The model under review builds one solid part; all positions refer to its coordinate system, in mm. A direction names the side the tool comes from. Coordinates: 2 decimals unless noted, no trailing zeros. Loops run counter-clockwise (first coordinate to the right, second up) from the corner with the lowest first, then second, coordinate; pieces in that order, holes last. Notation, with made-up numbers: M -29,-37 L 28,-37 A26 ccw 28,-22 Z; hole C -29.5,62 d6. An arc over 180 degrees is marked long. Return JSON: item names as keys, results as strings.
```python
from build123d import *

# Parameters (mm, degrees)
EXTRUSION1_DEPTH           = 6.6
EXTRUSION1_TAPER           = 4.000000000000009
EXTRUSION1_OTHER_WAY_DEPTH = 6.6
EXTRUSION1_OTHER_WAY_TAPER = 4.000000000000009
CONG_1_R                   = 1
ESQUISSE2_R                = 2.7
ENL_V_MAT_EXTRU_1_DEPTH    = 35.77427225377981
EXTRUSION2_START           = -11
EXTRUSION2_DEPTH           = 11
EXTRUSION3_DEPTH           = 19.5
ESQUISSE5_W                = 3.2474365518074073
ESQUISSE5_H                = 0.8522228738252646
ESQUISSE5_W_2              = 3.247436551807409
EXTRUSION4_DEPTH           = 5


with BuildPart() as part:
    # Esquisse1 → Extrusion1 (new body)
    with BuildSketch(Plane.XY):
        with BuildLine():
            Line((2.000000000000013, 0), (26.500000000000004, 0))
            ThreePointArc((26.500000000000004, 0), (27.9142135623731, 0.5857864376269051), (28.500000000000004, 2.0000000000000004))
            Line((28.500000000000004, 2.0000000000000004), (28.499999999999996, 16.8))
            ThreePointArc((28.499999999999996, 16.8), (27.914213562373096, 18.2142135623731), (26.499999999999996, 18.800000000000004))
            Line((26.499999999999996, 18.800000000000004), (2, 18.800000000000004))
            ThreePointArc((2, 18.800000000000004), (0.5857864376269051, 18.214213562373097), (0, 16.8))
            Line((0, 16.8), (-6.3e-16, 2.000000000000013))
            ThreePointArc((-6.3e-16, 2.000000000000013), (0.5857864376269053, 0.5857864376269042), (2.000000000000013, 0))
        make_face()
    extrude(amount=EXTRUSION1_DEPTH, taper=EXTRUSION1_TAPER)

    # Esquisse1 → Extrusion1 other way (add)
    with BuildSketch(Plane.XY):
        with BuildLine():
            Line((2.000000000000013, 0), (26.500000000000004, 0))
            ThreePointArc((26.500000000000004, 0), (27.9142135623731, 0.5857864376269051), (28.500000000000004, 2.0000000000000004))
            Line((28.500000000000004, 2.0000000000000004), (28.499999999999996, 16.8))
            ThreePointArc((28.499999999999996, 16.8), (27.914213562373096, 18.2142135623731), (26.499999999999996, 18.800000000000004))
            Line((26.499999999999996, 18.800000000000004), (2, 18.800000000000004))
            ThreePointArc((2, 18.800000000000004), (0.5857864376269051, 18.214213562373097), (0, 16.8))
            Line((0, 16.8), (-6.3e-16, 2.000000000000013))
            ThreePointArc((-6.3e-16, 2.000000000000013), (0.5857864376269053, 0.5857864376269042), (2.000000000000013, 0))
        make_face()
    extrude(amount=-EXTRUSION1_OTHER_WAY_DEPTH, taper=EXTRUSION1_OTHER_WAY_TAPER)

    # Congé1
    cong_1_edges = [part.edges().sort_by_distance(p)[0] for p in [
        (0.9121282088461893, 0.9121282088461893, 6.6),
        (14.250000000000007, 0.46151695882717014, 6.6000000000000005),
        (27.587871791153816, 0.9121282088461893, 6.6),
        (28.03848304117283, 9.4, 6.6000000000000005),
        (27.587871791153812, 17.887871791153817, 6.6),
        (14.25, 18.338483041172836, 6.6000000000000005),
        (0.9121282088461911, 17.887871791153813, -6.6),
        (14.250000000000005, 18.338483041172836, -6.6),
        (27.587871791153812, 17.887871791153813, -6.6),
        (28.03848304117283, 9.400000000000006, -6.6),
        (27.587871791153816, 0.9121282088461875, -6.6),
        (14.250000000000004, 0.46151695882717014, -6.6),
        (0.9121282088461893, 0.9121282088461893, -6.6),
        (0.46151695882717014, 9.4, -6.6),
        (0.9121282088461893, 17.887871791153813, 6.6),
        (0.46151695882717014, 9.400000000000006, 6.6000000000000005),
    ]]
    fillet(cong_1_edges, radius=CONG_1_R)

    # Esquisse2 → Enlèv. mat.-Extru.1 (cut, through all)
    with BuildSketch(Plane(origin=(0, 0, 0), x_dir=(0, 0, -1), z_dir=(1, 0, 0))):
        with Locations(Location((0, 9.40000000000001, 0), (0, 0, 90))):
            Circle(ESQUISSE2_R)
    extrude(amount=ENL_V_MAT_EXTRU_1_DEPTH, mode=Mode.SUBTRACT)

    # Esquisse3 → Extrusion2 (add)
    with BuildSketch(Plane(origin=(10, 0, 0), x_dir=(0, 0, -1), z_dir=(1, 0, 0)).offset(EXTRUSION2_START)):
        with BuildLine():
            ThreePointArc((0, 12.100000000000007), (-2.6999999999999975, 9.400000000000007), (6.16e-15, 6.700000000000009))
            ThreePointArc((6.16e-15, 6.700000000000009), (0.5000000000000038, 6.200000000000009), (5.89e-15, 5.700000000000011))
            ThreePointArc((5.89e-15, 5.700000000000011), (-3.6999999999999975, 9.400000000000006), (2.3e-16, 13.100000000000007))
            ThreePointArc((2.3e-16, 13.100000000000007), (0.4999999999999991, 12.600000000000007), (0, 12.100000000000007))
        make_face()
    extrude(amount=EXTRUSION2_DEPTH)

    # Esquisse4 → Extrusion3 (add)
    with BuildSketch(Plane(origin=(10, 0, 0), x_dir=(0, 0, -1), z_dir=(1, 0, 0))):
        with BuildLine():
            ThreePointArc((0, 6.700000000000006), (2.700000000000003, 9.400000000000043), (-6.772e-14, 12.10000000000001))
            ThreePointArc((-6.772e-14, 12.10000000000001), (-0.5000000000000799, 12.6), (-9.088e-14, 13.10000000000001))
            ThreePointArc((-9.088e-14, 13.10000000000001), (3.700000000000002, 9.400000000000054), (-6.8e-16, 5.700000000000007))
            ThreePointArc((-6.8e-16, 5.700000000000007), (-0.5000000000000002, 6.200000000000007), (0, 6.700000000000006))
        make_face()
    extrude(amount=EXTRUSION3_DEPTH)

    # Esquisse5 → Extrusion4 (cut)
    with BuildSketch(Plane.XY.offset(6.6)):
        with Locations((20.306831390499674, 1.820143481877461)):
            Rectangle(ESQUISSE5_W, ESQUISSE5_H)
        with Locations((8.193168609500333, 1.820143481877461)):
            Rectangle(ESQUISSE5_W_2, ESQUISSE5_H)
        Polygon((1.7379562995508964, 14.367502834636706), (4.041510066838186, 17.227086821613987), (4.636308888649757, 16.74794332626577), (2.3327551213624673, 13.888359339288488), align=None)
        Polygon((2.3327551213624673, 4.911640660711529), (4.636308888649757, 2.052056673734249), (4.041510066838186, 1.5729131783860304), (1.7379562995508964, 4.432497165363312), align=None)
        Polygon((26.762043700449112, 4.43249716536331), (24.45848993316182, 1.5729131783860304), (23.863691111350253, 2.0520566737342487), (26.16724487863754, 4.9116406607115275), align=None)
        Polygon((26.16724487863754, 13.888359339288483), (23.863691111350253, 16.747943326265762), (24.45848993316182, 17.227086821613973), (26.762043700449112, 14.3675028346367), align=None)
    extrude(amount=-EXTRUSION4_DEPTH, mode=Mode.SUBTRACT)


solid = part.part
```
1. Add section B-B on z = -2. Give the boundary of the cut face in (x, y), plus the area to 3 significant figures.
Check values:
{"outline": "M 0.14,2 A1.86 ccw 2,0.14 L 26.5,0.14 A1.86 ccw 28.36,2 L 28.36,6.29 L 29.5,6.29 L 29.5,7.59 L 0.14,7.59 Z; M 0.14,11.21 L 29.5,11.21 L 29.5,12.51 L 28.36,12.51 L 28.36,16.8 A1.86 ccw 26.5,18.66 L 2,18.66 A1.86 ccw 0.14,16.8 Z", "area": "420 mm²"}
2. Add section A-A on x = 17.5. Give the boundary of the cut face in (y, z).
Check values:
{"outline": "M 0,0 L 0.4,-5.67 A1 ccw 1.39,-6.6 L 17.41,-6.6 A1 ccw 18.4,-5.67 L 18.8,0 L 18.4,5.67 A1 ccw 17.41,6.6 L 1.39,6.6 A1 ccw 0.4,5.67 Z; hole C 9.4,0 d5.4"}
3. Add section D-D on y = 12.5. Give the boundary of the cut face in (x, z).
Check values:
{"outline": "M -1,-0.49 L 0.03,-0.49 L 0.4,-5.67 A1 ccw 1.39,-6.6 L 27.11,-6.6 A1 ccw 28.1,-5.67 L 28.36,-2.02 L 29.5,-2.02 L 29.5,0.49 L 28.47,0.49 L 28.1,5.67 A1 ccw 27.11,6.6 L 1.39,6.6 A1 ccw 0.4,5.67 L 0.14,2.02 L -1,2.02 Z"}
4. The part is to be moulded in two halves that separate along X. For faces 1 (the face through (27.786, 18.058, -2.875)), 2 (the face through (3.5, 15.34, 4.14)), 3 (the face through (14.08, 18.08, -6.34)), say which applies: released by +X, released by -X, zero draft, split by the parting line, or undercut.
Check values:
{"face 1": "released by +X", "face 2": "undercut", "face 3": "zero draft"}
5. Insertion check: pin 1 Ø0.7 at (y, z) = (2, 3) entering from -X; pin 2 Ø0.7 at (y, z) = (2, 3.5) entering from +X; pin 3 Ø1.5 at (y, z) = (14.5, 1.5) entering from -X. Each pin has a flat end and moves straight along its axis. Give the tip position at first contact, or say it passes through.
Check values:
{"pin 1": "x = 0.19", "pin 2": "x = 28.28", "pin 3": "x = 0.05"}
6. Machinability: for faces 4 (the face through (29, 9.5, -3.7)), 5 (the face through (-1, 9, 3)), 6 (the face through (0.284, 9.296, 4.055)), 7 (the face through (14, 10, -6.6)), 8 (the face through (25, 3, 1.6)), which of the approach directions +Z, -Z, +X, -X, +Y, -Y give a long, thin tool a straight path to every point of the face, cutting with its end or side? Answer none if there is none.
Check values:
{"face 4": "-Z, +X", "face 5": "+Z, -Z, -X, +Y, -Y", "face 6": "+Z, -X", "face 7": "-Z, +X, -X, +Y, -Y", "face 8": "+Z"}
7. Add section C-C on y = 9.4. Give the boundary of the cut face in (x, z).
Check values:
{"outline": "M -1,2.7 L 28.31,2.7 L 28.1,5.67 A1 ccw 27.11,6.6 L 1.39,6.6 A1 ccw 0.4,5.67 L 0.26,3.7 L -1,3.7 Z; M 0.19,-2.7 L 0.4,-5.67 A1 ccw 1.39,-6.6 L 27.11,-6.6 A1 ccw 28.1,-5.67 L 28.24,-3.7 L 29.5,-3.7 L 29.5,-2.7 Z"}
8. To check wall thickness, follow line 1 (Z direction, x = 14.5, y = 9.4); line 2 (Y direction, x = 18, z = 0); line 3 (Y direction, x = 4.5, z = 5). State the ranges of each line that lie inside material, in increasing order.
Check values:
{"line 1": "-6.6 to -2.7, 2.7 to 6.6", "line 2": "0 to 6.7, 12.1 to 18.8", "line 3": "0.35 to 1.94, 2.22 to 16.58, 16.86 to 18.45"}
